```python
from build123d import *

# Parameters (mm, degrees)
BOSS_EXTRUDE2_DEPTH      = 10
BOSS_EXTRUDE3_DEPTH      = 20
BOSS_EXTRUDE3_DEPTH_BACK = 30
SKETCH4_R                = 15
CUT_EXTRUDE1_DEPTH       = 51
SKETCH5_W                = 25
SKETCH5_H                = 9
BOSS_EXTRUDE4_DEPTH      = 15
BOSS_EXTRUDE5_DEPTH      = 9
BOSS_EXTRUDE6_DEPTH      = 9
SKETCH8_R                = 6
CUT_EXTRUDE2_DEPTH       = 46


with BuildPart() as part:
    # Sketch1 → Boss-Extrude2 (new body)
    with BuildSketch(Plane(origin=(0, 0, 0), x_dir=(1, 0, 0), z_dir=(0, 1, 0))):
        with BuildLine():
            Line((-9.01734104, 28.612716763), (-97.5, 15))
            Line((-97.5, 15), (-122.5, 15))
            Line((-122.5, 15), (-122.5, -15))
            Line((-122.5, -15), (-97.5, -15))
            Line((-97.5, -15), (-9.01734104, -28.612716763))
            ThreePointArc((-9.01734104, -28.612716763), (-30, 0), (-9.01734104, 28.612716763))
        make_face()
        with BuildLine():
            Line((0, 30), (-9.01734104, 28.612716763))
            ThreePointArc((-9.01734104, 28.612716763), (-30, 0), (-9.01734104, -28.612716763))
            Line((-9.01734104, -28.612716763), (0, -30))
            ThreePointArc((0, -30), (21.213203436, -21.213203436), (30, 0))
            ThreePointArc((30, 0), (21.213203436, 21.213203436), (0, 30))
        make_face()
    extrude(amount=BOSS_EXTRUDE2_DEPTH)

    # Sketch3 → Boss-Extrude3 (add, two sides)
    with BuildSketch(Plane(origin=(0, 10, 0), x_dir=(1, 0, 0), z_dir=(0, 1, 0))) as boss_extrude3_sk:
        with BuildLine():
            Line((0, 30), (-9.01734104, 28.612716763))
            ThreePointArc((-9.01734104, 28.612716763), (-30, 0), (-9.01734104, -28.612716763))
            Line((-9.01734104, -28.612716763), (0, -30))
            ThreePointArc((0, -30), (21.213203436, -21.213203436), (30, 0))
            ThreePointArc((30, 0), (21.213203436, 21.213203436), (0, 30))
        make_face()
    extrude(amount=BOSS_EXTRUDE3_DEPTH)
    extrude(boss_extrude3_sk.sketch, amount=-BOSS_EXTRUDE3_DEPTH_BACK)

    # Sketch4 → Cut-Extrude1 (cut, through all)
    with BuildSketch(Plane(origin=(0, 30, 0), x_dir=(1, 0, 0), z_dir=(0, 1, 0))):
        Circle(SKETCH4_R)
    extrude(amount=-CUT_EXTRUDE1_DEPTH, mode=Mode.SUBTRACT)

    # Sketch5 → Boss-Extrude4 (add)
    with BuildSketch(Plane(origin=(0, 10, 0), x_dir=(1, 0, 0), z_dir=(0, 1, 0))):
        with Locations((-110, 10.5)):
            Rectangle(SKETCH5_W, SKETCH5_H)
        with Locations((-110, -10.5)):
            Rectangle(SKETCH5_W, SKETCH5_H)
    extrude(amount=BOSS_EXTRUDE4_DEPTH)

    # Sketch6 → Boss-Extrude5 (add)
    with BuildSketch(Plane.XY.offset(15)):
        with BuildLine():
            ThreePointArc((-122.5, 25), (-110, 37.5), (-97.5, 25))
            Line((-97.5, 25), (-122.5, 25))
        make_face()
    extrude(amount=-BOSS_EXTRUDE5_DEPTH)

    # Sketch7 → Boss-Extrude6 (add)
    with BuildSketch(Plane(origin=(0, 0, -15), x_dir=(-1, 0, 0), z_dir=(0, 0, -1))):
        with BuildLine():
            Line((97.5, 25), (122.5, 25))
            ThreePointArc((122.5, 25), (110, 37.5), (97.5, 25))
        make_face()
    extrude(amount=-BOSS_EXTRUDE6_DEPTH)

    # Sketch8 → Cut-Extrude2 (cut, through all)
    with BuildSketch(Plane.XY.offset(15)):
        with Locations((-110, 25)):
            Circle(SKETCH8_R)
    extrude(amount=-CUT_EXTRUDE2_DEPTH, mode=Mode.SUBTRACT)


solid = part.part
```
Build history of the part. All positions in model axes, mm. A direction names the side the tool comes from. Coordinates: 2 decimals unless noted, no trailing zeros. Order: outer loops, then holes, each group sorted by start corner. A loop starts at its lowest first (then second) coordinate and runs counter-clockwise, first axis right, second up. Notation, with made-up numbers: (30, 12.25) -> (44, 12.25) arc R25 cw to (44, 35.25) -> close; hole circle Ø5 at (0, 85.25). An arc over 180 degrees is marked (long way). Answer in a Markdown table with one row per item. Add a question column.
Q1. Band-saw the part on C-C, the plane z = -13.5. List the corners of the cut face in (x, y).
Q2. Band-saw the part on D-D, the plane x = 7. List the corners of the cut face in (y, z).
Q3. Band-saw the part on B-B, the plane y = 13. List the corners of the cut face in (x, z), then the cut area to 3 significant figures.
Q4. Wall check: line 1 along X through (y, z) = (23.5, 10); line 2 along Y through (x, z) = (-110, 9.75); line 3 along X through (y, z) = (10.5, 10). Give the ranges that are in metal, low to high. Write a range as [from, to].
Q5. Which spindle directions (+Z, -Z, +X, -X, +Y, -Y) get a long thin tool onto all of the face, cutting with end or side? Do faces 4 (the face through (6, 30, -14)), 5 (the face through (-67, 10, 0)), 6 (the face through (-97.5, 17, 11)), 7 (the face through (-110, 15, 15)), 8 (the face through (-110, 18, 6)). Say none if no direction does.
Q6. Band-saw the part on A-A, the plane x = -110. List the corners of the cut face in (y, z), then the cut area to 3 significant figures.
Q7. Mould opens along X. For faces 1 (the face through (-29.995, -9.86, -0.531)), 2 (the face through (-29.995, 19.86, -0.531)), 3 (the face through (-110, 15, -15)) say: +X half, -X half, draft (parallel to the pull), parting line (faces both ways), or undercut.
Q8. Drop flat-ended pins along their axis: pin 1 (10 mm diameter, centred on x = -50, z = 23.5, fed in from -Y); pin 2 (12.5 mm diameter, centred on x = -115.5, y = 22, fed in from +Z); pin 3 (7.5 mm diameter, centred on x = -108.5, y = 30, fed in from -Z). Give the stop position or say it passes through.
Answers follow:
| question | item | result |
|---|---|---|
| 1 | outline | (-122.5, 0) -> (-26.79, 0) -> (-26.79, -20) -> (-6.54, -20) -> (-6.54, 30) -> (-26.79, 30) -> (-26.79, 10) -> (-97.5, 10) -> (-97.5, 25) arc R12.5 ccw to (-122.5, 25) -> close; (6.54, -20) -> (26.79, -20) -> (26.79, 30) -> (6.54, 30) -> close; hole circle Ø12 at (-110, 25) |
| 2 | outline | (-20, -29.17) -> (30, -29.17) -> (30, -13.27) -> (-20, -13.27) -> close; (-20, 13.27) -> (30, 13.27) -> (30, 29.17) -> (-20, 29.17) -> close |
| 3 | outline | (-122.5, -15) -> (-97.5, -15) -> (-97.5, -6) -> (-122.5, -6) -> close; (-122.5, 6) -> (-97.5, 6) -> (-97.5, 15) -> (-122.5, 15) -> close; (-9.02, -28.61) -> (0, -30) arc R30 ccw to (0, 30) -> (-9.02, 28.61) arc R30 ccw to start; hole circle Ø30 at (0, 0) |
| 3 | area | 2,570 mm^2 |
| 4 | line 1 | [-122.5, -115.81], [-104.19, -97.5], [-28.28, -11.18], [11.18, 28.28] |
| 4 | line 2 | [0, 19], [31, 37.5] |
| 4 | line 3 | [-122.5, -97.5], [-28.28, -11.18], [11.18, 28.28] |
| 5 | face 4 | +Z, -Z, +X, +Y |
| 5 | face 5 | +Y |
| 5 | face 6 | +Z, -Z, +Y |
| 5 | face 7 | +Z, -X, +Y, -Y |
| 5 | face 8 | -X, +Y |
| 6 | outline | (0, -15) -> (19, -15) -> (19, -6) -> (10, -6) -> (10, 6) -> (19, 6) -> (19, 15) -> (0, 15) -> close; (31, -15) -> (37.5, -15) -> (37.5, -6) -> (31, -6) -> close; (31, 6) -> (37.5, 6) -> (37.5, 15) -> (31, 15) -> close |
| 6 | area | 579 mm^2 |
| 7 | face 1 | -X half |
| 7 | face 2 | undercut |
| 7 | face 3 | draft |
| 8 | pin 1 | y = 0 |
| 8 | pin 2 | z = 15 |
| 8 | pin 3 | z = -15 |
